```python
from build123d import *

# Parameters (mm, degrees)
BOSS_EXTRUDE1_DEPTH     = 6.35
SKETCH2_W               = 63.5
SKETCH2_H               = 34.925
CUT_EXTRUDE1_DEPTH      = 299.126542166
F_1_4_CLEARANCE_HOLE1_D = 6.7564
CUT_EXTRUDE2_DEPTH      = 299.126542166
FILLET1_R               = 25.4
FILLET2_R               = 5.08
FILLET3_R               = 2.54
CUT_EXTRUDE4_DEPTH      = 276.239678724
FILLET5_R               = 12.7
FILLET6_R               = 38.1


with BuildPart() as part:
    # Sketch1 → Boss-Extrude1 (new body)
    with BuildSketch(Plane(origin=(0, 0, 0), x_dir=(1, 0, 0), z_dir=(0, 1, 0))):
        with BuildLine():
            Line((22.225, 228.6), (-22.225, 228.6))
            Line((-22.225, 228.6), (-22.225, 190.5))
            ThreePointArc((-22.225, 190.5), (-25.761770597, 174.46899338), (-35.715455289, 161.414259351))
            Line((-35.715455289, 161.414259351), (-168.508098746, 49.057949228))
            ThreePointArc((-168.508098746, 49.057949228), (-185.296646926, 27.038964499), (-191.262, 0))
            Line((-191.262, 0), (-191.262, -3.175))
            Line((-191.262, -3.175), (-153.162, -3.175))
            Line((-153.162, -3.175), (-153.162, 0))
            ThreePointArc((-153.162, 0), (-127, 26.162), (-100.838, 0))
            Line((-100.838, 0), (-100.838, -3.175))
            Line((-100.838, -3.175), (100.838, -3.175))
            Line((100.838, -3.175), (100.838, 0))
            ThreePointArc((100.838, 0), (127, 26.162), (153.162, 0))
            Line((153.162, 0), (153.162, -3.175))
            Line((153.162, -3.175), (191.262, -3.175))
            Line((191.262, -3.175), (191.262, 0))
            ThreePointArc((191.262, 0), (185.296646926, 27.038964499), (168.508098746, 49.057949228))
            Line((168.508098746, 49.057949228), (35.715455289, 161.414259351))
            ThreePointArc((35.715455289, 161.414259351), (25.761770597, 174.46899338), (22.225, 190.5))
            Line((22.225, 190.5), (22.225, 228.6))
        make_face()
    extrude(amount=BOSS_EXTRUDE1_DEPTH)

    # Sketch2 → Cut-Extrude1 (cut, through all)
    with BuildSketch(Plane(origin=(0, 6.35, 0), x_dir=(1, 0, 0), z_dir=(0, 1, 0))):
        with Locations((0, 14.2875)):
            Rectangle(SKETCH2_W, SKETCH2_H)
    extrude(amount=-CUT_EXTRUDE1_DEPTH, mode=Mode.SUBTRACT)

    # 1/4 Clearance Hole1 (through all)
    with Locations(Plane(origin=(0, 6.35, 0), x_dir=(1, 0, 0), z_dir=(0, 1, 0))):
        with Locations((0, 209.55), (0, 133.35), (0, 57.15)):
            Hole(F_1_4_CLEARANCE_HOLE1_D / 2)

    # Sketch5 → Cut-Extrude2 (cut, through all)
    with BuildSketch(Plane(origin=(0, 6.35, 0), x_dir=(1, 0, 0), z_dir=(0, 1, 0))):
        with BuildLine():
            Line((-153.162, -3.175), (-153.162, 62.042335901))
            Line((-153.162, 62.042335901), (-168.508098746, 49.057949228))
            ThreePointArc((-168.508098746, 49.057949228), (-185.296646926, 27.038964499), (-191.262, 0))
            Line((-191.262, 0), (-191.262, -3.175))
            Line((-191.262, -3.175), (-153.162, -3.175))
        make_face()
        with BuildLine():
            Line((191.262, 0), (191.262, -3.175))
            Line((191.262, -3.175), (153.162, -3.175))
            Line((153.162, -3.175), (153.162, 62.042335901))
            Line((153.162, 62.042335901), (168.508098746, 49.057949228))
            ThreePointArc((168.508098746, 49.057949228), (185.296646926, 27.038964499), (191.262, 0))
        make_face()
    extrude(amount=-CUT_EXTRUDE2_DEPTH, mode=Mode.SUBTRACT)

    # Fillet1
    fillet1_edges = [part.edges().sort_by_distance(p)[0] for p in [
        (153.162, 3.175, -62.042335901),
        (-153.162, 3.175, -62.042335901),
    ]]
    fillet(fillet1_edges, radius=FILLET1_R)

    # Fillet2
    fillet2_edges = [part.edges().sort_by_distance(p)[0] for p in [
        (153.162, 3.175, 0),
        (-153.162, 3.175, 0),
    ]]
    fillet(fillet2_edges, radius=FILLET2_R)

    # Fillet3
    fillet3_edges = [part.edges().sort_by_distance(p)[0] for p in [
        (-22.225, 3.175, -228.6),
        (22.225, 3.175, -228.6),
        (100.838, 3.175, 3.175),
        (-100.838, 3.175, 3.175),
        (31.75, 3.175, 3.175),
        (-31.75, 3.175, 3.175),
        (-31.75, 3.175, -31.75),
        (31.75, 3.175, -31.75),
    ]]
    fillet(fillet3_edges, radius=FILLET3_R)

    # Sketch7 → Cut-Extrude4 (cut, through all)
    with BuildSketch(Plane(origin=(0, 6.35, 0), x_dir=(1, 0, 0), z_dir=(0, 1, 0))):
        Polygon((-22.225, 125.857901259), (-153.162, 50.261389063), (-153.162, 60.856337773), (-22.225, 190.5), align=None)
        Polygon((153.162, 60.856337773), (153.162, 50.261389063), (22.225, 125.857901259), (22.225, 190.5), align=None)
    extrude(amount=-CUT_EXTRUDE4_DEPTH, mode=Mode.SUBTRACT)

    # Fillet5
    fillet5_edges = [part.edges().sort_by_distance(p)[0] for p in [
        (153.162, 3.175, -50.261389063),
        (-153.162, 3.175, -50.261389063),
    ]]
    fillet(fillet5_edges, radius=FILLET5_R)

    # Fillet6
    fillet6_edges = [part.edges().sort_by_distance(p)[0] for p in [
        (-22.225, 3.175, -125.857901259),
        (22.225, 3.175, -125.857901259),
    ]]
    fillet(fillet6_edges, radius=FILLET6_R)


solid = part.part
```
Work out the finished part from the listing and answer in its coordinate system (mm). A direction names the side the tool comes from. Coordinates: 2 decimals unless noted, no trailing zeros. Loops run counter-clockwise (first coordinate to the right, second up) from the corner with the lowest first, then second, coordinate; pieces in that order, holes last. Notation, with made-up numbers: (-20.5, 64.5) -> (8.5, 64.5) arc R22 cw to (8.5, 84.5) -> close; hole circle Ø8 at (-31, 15.5). An arc over 180 degrees is marked (long way). Answer as CSV lines item,"result".
Q1. Find the intervals of material crossed by probe 1 along Z at (x, y) = (0, 3.75); probe 2 along X at (y, z) = (2.75, -209.55) (3 decimals); probe 3 along X at (y, z) = (3, -149) (3 decimals), in increasing order.
Findings:
probe 1,"z = -228.6 to -212.93, -206.17 to -136.73, -129.97 to -60.53, -53.77 to -31.75"
probe 2,"x = -22.225 to -3.378, 3.378 to 22.225"
probe 3,"x = -22.225 to 22.225"
Q2. For a pull along X with two mould halves and no side action, classify faces 3 (the face through (-2, 0, -63)), 4 (the face through (-151.507, 3.131, -49.198)), 5 (the face through (116.064, 3.131, -23.767)), 6 (the face through (151.414, 3.131, -49.359)) as +X half, -X half, draft (parallel to the pull), parting line (faces both ways), or undercut.
Findings:
face 3,"draft"
face 4,"-X half"
face 5,"undercut"
face 6,"+X half"
Q3. The part is cut by section C-C on y = 4. State how many separate pieces and enclosed holes the cut face has, and give its area (3 significant figures).
Findings:
separate pieces,"1"
enclosed holes,"3"
area,"29,400 mm²"
Q4. A tool of negligible diameter and unlimited length cuts with its end or side. For faces 1 (the face through (-31.75, 3, -14)), 2 (the face through (-27.19, 3.13, -129.05)), from which of +Z, -Z, +X, -X, +Y, -Y can it reach the whole face along a straight path? Write none if from no direction.
Findings:
face 1,"+Z, +Y, -Y"
face 2,"-Z, -X, +Y, -Y"
Q5. The part is cut by section A-A on z = -209.55. Write down the section's boundary in (x, y) (3 decimals), and give its area (3 significant figures).
Findings:
outline,"(-22.225, 0) -> (-3.378, 0) -> (-3.378, 6.35) -> (-22.225, 6.35) -> close; (3.378, 0) -> (22.225, 0) -> (22.225, 6.35) -> (3.378, 6.35) -> close"
area,"239 mm²"
Q6. Each of these flat-tipped pins is pushed along its axis until it touches: pin 1 (3 mm diameter, centred on y = 3.5, z = -195, fed in from +X) (3 decimals); pin 2 (0.5 mm diameter, centred on y = 4, z = 0, fed in from +X); pin 3 (2 mm diameter, centred on x = -96, y = 4, fed in from -Z); pin 4 (5 mm diameter, centred on x = -107.5, z = -32.5, fed in from -Y). Where does it stop, or does it pass through?
Findings:
pin 1,"stops at x = 22.225"
pin 2,"stops at x = 100.84"
pin 3,"stops at z = -83.84"
pin 4,"stops at y = 0"
Q7. The part is cut by section D-D on z = -57.15. Write down the section's boundary in (x, y).
Findings:
outline,"(-141.23, 0) -> (-3.38, 0) -> (-3.38, 6.35) -> (-141.23, 6.35) -> close; (3.38, 0) -> (141.23, 0) -> (141.23, 6.35) -> (3.38, 6.35) -> close"
Q8. The part is cut by section B-B on x = 0. Write down the section's boundary in (y, z).
Findings:
outline,"(0, -228.6) -> (6.35, -228.6) -> (6.35, -212.93) -> (0, -212.93) -> close; (0, -206.17) -> (6.35, -206.17) -> (6.35, -136.73) -> (0, -136.73) -> close; (0, -129.97) -> (6.35, -129.97) -> (6.35, -60.53) -> (0, -60.53) -> close; (0, -53.77) -> (6.35, -53.77) -> (6.35, -31.75) -> (0, -31.75) -> close"
